from build123d import *

# Parameters (mm, degrees)
SKETCH1_W                       = 46
SKETCH1_H                       = 32
BOSS_EXTRUDE1_DEPTH             = 2
CBORE_FOR_M3_SBHCS1_AT_2_COUNT  = 2
CBORE_FOR_M3_SBHCS1_AT_2_PITCH  = 18.273746641
CBORE_FOR_M3_SBHCS1_AT_3_COUNT  = 2
CBORE_FOR_M3_SBHCS1_AT_3_PITCH  = 37.721741957
CBORE_FOR_M3_SBHCS1_AT_4_COUNT  = 2
CBORE_FOR_M3_SBHCS1_AT_4_PITCH  = 33
BOSS_EXTRUDE2_START             = 3.63
SKETCH9_R                       = 3.35
SKETCH9_R_2                     = 1.7
BOSS_EXTRUDE2_DEPTH             = 3.63
SKETCH11_R                      = 5
SKETCH11_R_2                    = 3
BOSS_EXTRUDE3_DEPTH             = 2
CBORE_FOR_M1_6_SHCS1_AT_2_COUNT = 2
CBORE_FOR_M1_6_SHCS1_AT_2_PITCH = 33.25
CBORE_FOR_M1_6_SHCS1_AT_3_COUNT = 2
CBORE_FOR_M1_6_SHCS1_AT_3_PITCH = 51.03253864
CBORE_FOR_M1_6_SHCS1_AT_4_COUNT = 2
CBORE_FOR_M1_6_SHCS1_AT_4_PITCH = 28.4
CUT_EXTRUDE1_START              = -2
SKETCH17_R                      = 3
CUT_EXTRUDE1_DEPTH              = 2
FILLET1_R                       = 1.5
SKETCH18_W                      = 2
SKETCH18_H                      = 24
BOSS_EXTRUDE4_DEPTH             = 17.5
SKETCH19_R                      = 1.215
SKETCH19_R_2                    = 1.22
BOSS_EXTRUDE5_DEPTH             = 17.5


with BuildPart() as part:
    # Sketch1 → Boss-Extrude1 (new body)
    with BuildSketch(Plane(origin=(0, 0, 0), x_dir=(1, 0, 0), z_dir=(0, 1, 0))):
        with Locations((-23, -16)):
            Rectangle(SKETCH1_W, SKETCH1_H)
    extrude(amount=BOSS_EXTRUDE1_DEPTH)

    # Sketch7 → CBORE for M3 SBHCS1 (revolve, cut)
    with BuildSketch(Plane(origin=(-39.5, 2, 6.726253359), x_dir=(0, 0, 1), z_dir=(1, 0, 0))):
        Polygon((0, 0), (0, 3.021463052), (1.7, 2), (1.7, 1.65), (3.35, 1.65), (3.35, 0.025), (3.375, 0), align=None)
    cbore_for_m3_sbhcs1 = revolve(axis=Axis((-39.5, 8.35, 6.726253359), (0, -1, 0)), mode=Mode.SUBTRACT)

    # CBORE for M3 SBHCS1 at 2: CBORE for M3 SBHCS1 ×2
    with Locations(*[(0, 0, i * CBORE_FOR_M3_SBHCS1_AT_2_PITCH) for i in range(1, CBORE_FOR_M3_SBHCS1_AT_2_COUNT)]):
        add(cbore_for_m3_sbhcs1, mode=Mode.SUBTRACT)

    # CBORE for M3 SBHCS1 at 3: CBORE for M3 SBHCS1 ×2
    with Locations(*[Vector(0.874827043707974, 0, 0.4844353864006702) * (i * CBORE_FOR_M3_SBHCS1_AT_3_PITCH) for i in range(1, CBORE_FOR_M3_SBHCS1_AT_3_COUNT)]):
        add(cbore_for_m3_sbhcs1, mode=Mode.SUBTRACT)

    # CBORE for M3 SBHCS1 at 4: CBORE for M3 SBHCS1 ×2
    with Locations(*[(i * CBORE_FOR_M3_SBHCS1_AT_4_PITCH, 0, 0) for i in range(1, CBORE_FOR_M3_SBHCS1_AT_4_COUNT)]):
        add(cbore_for_m3_sbhcs1, mode=Mode.SUBTRACT)

    # Sketch9 → Boss-Extrude2 (add)
    # profile 1 of 4: a face of its own
    with BuildSketch(Plane(origin=(-49.887058416, 0.35, -0.273746641), x_dir=(1, 0, 0), z_dir=(0, 1, 0)).offset(BOSS_EXTRUDE2_START)):
        with Locations(Location((10.387058416, -25.273746641, 0), (0, 0, 90))):
            Circle(SKETCH9_R)
        with Locations(Location((10.387058416, -25.273746641, 0), (0, 0, 270))):
            Circle(SKETCH9_R_2, mode=Mode.SUBTRACT)
    # profile 2 of 4: a face of its own
    with BuildSketch(Plane(origin=(-49.887058416, 0.35, -0.273746641), x_dir=(1, 0, 0), z_dir=(0, 1, 0)).offset(BOSS_EXTRUDE2_START)):
        with Locations(Location((43.387058416, -25.273746641, 0), (0, 0, 90))):
            Circle(SKETCH9_R)
        with Locations(Location((43.387058416, -25.273746641, 0), (0, 0, 270))):
            Circle(SKETCH9_R_2, mode=Mode.SUBTRACT)
    # profile 3 of 4: a face of its own
    with BuildSketch(Plane(origin=(-49.887058416, 0.35, -0.273746641), x_dir=(1, 0, 0), z_dir=(0, 1, 0)).offset(BOSS_EXTRUDE2_START)):
        with Locations(Location((43.387058416, -7, 0), (0, 0, 90))):
            Circle(SKETCH9_R)
        with Locations(Location((43.387058416, -7, 0), (0, 0, 270))):
            Circle(SKETCH9_R_2, mode=Mode.SUBTRACT)
    # profile 4 of 4: a face of its own
    with BuildSketch(Plane(origin=(-49.887058416, 0.35, -0.273746641), x_dir=(1, 0, 0), z_dir=(0, 1, 0)).offset(BOSS_EXTRUDE2_START)):
        with Locations(Location((10.387058416, -7, 0), (0, 0, 90))):
            Circle(SKETCH9_R)
        with Locations(Location((10.387058416, -7, 0), (0, 0, 270))):
            Circle(SKETCH9_R_2, mode=Mode.SUBTRACT)
    extrude(amount=-BOSS_EXTRUDE2_DEPTH)

    # Sketch11 → Boss-Extrude3 (add)
    with BuildSketch(Plane(origin=(-49.887058416, 2, -0.273746641), x_dir=(1, 0, 0), z_dir=(0, 1, 0))):
        with Locations(Location((19.387058416, -16, 0), (0, 0, 270))):
            Circle(SKETCH11_R)
        with Locations(Location((19.387058416, -16, 0), (0, 0, 270))):
            Circle(SKETCH11_R_2, mode=Mode.SUBTRACT)
    extrude(amount=BOSS_EXTRUDE3_DEPTH)

    # Sketch16 → CBORE for M1.6 SHCS1 (revolve, cut)
    with BuildSketch(Plane(origin=(-44.2, 2, 1.8), x_dir=(0, 0, 1), z_dir=(1, 0, 0))):
        Polygon((0, 0), (0, 2), (0.9, 2), (0.9, 1.6), (1.75, 1.6), (1.75, 0.025), (1.775, 0), align=None)
    cbore_for_m1_6_shcs1 = revolve(axis=Axis((-44.2, 8.35, 1.8), (0, -1, 0)), mode=Mode.SUBTRACT)

    # CBORE for M1.6 SHCS1 at 2: CBORE for M1.6 SHCS1 ×2
    with Locations(*[(i * CBORE_FOR_M1_6_SHCS1_AT_2_PITCH, 0, 0) for i in range(1, CBORE_FOR_M1_6_SHCS1_AT_2_COUNT)]):
        add(cbore_for_m1_6_shcs1, mode=Mode.SUBTRACT)

    # CBORE for M1.6 SHCS1 at 3: CBORE for M1.6 SHCS1 ×2
    with Locations(*[Vector(0.8308424611100395, 0, 0.5565076862152155) * (i * CBORE_FOR_M1_6_SHCS1_AT_3_PITCH) for i in range(1, CBORE_FOR_M1_6_SHCS1_AT_3_COUNT)]):
        add(cbore_for_m1_6_shcs1, mode=Mode.SUBTRACT)

    # CBORE for M1.6 SHCS1 at 4: CBORE for M1.6 SHCS1 ×2
    with Locations(*[(0, 0, i * CBORE_FOR_M1_6_SHCS1_AT_4_PITCH) for i in range(1, CBORE_FOR_M1_6_SHCS1_AT_4_COUNT)]):
        add(cbore_for_m1_6_shcs1, mode=Mode.SUBTRACT)

    # Sketch17 → Cut-Extrude1 (cut)
    with BuildSketch(Plane(origin=(0, 2, 0), x_dir=(1, 0, 0), z_dir=(0, 1, 0)).offset(CUT_EXTRUDE1_START)):
        with Locations(Location((-30.5, -15.726253359, 0), (0, 0, 270))):
            Circle(SKETCH17_R)
    extrude(amount=CUT_EXTRUDE1_DEPTH, mode=Mode.SUBTRACT)

    # Fillet1
    fillet1_edges = [part.edges().sort_by_distance(p)[0] for p in [
        (0, 1, 32),
        (0, 1, 0),
        (-46, 1, 0),
        (-46, 1, 32),
    ]]
    fillet(fillet1_edges, radius=FILLET1_R)

    # Sketch18 → Boss-Extrude4 (add)
    with BuildSketch(Plane.XZ):
        with Locations((-45, 16)):
            Rectangle(SKETCH18_W, SKETCH18_H)
    extrude(amount=BOSS_EXTRUDE4_DEPTH)

    # Sketch19 → Boss-Extrude5 (add)
    with BuildSketch(Plane.XZ):
        with Locations(Location((-18.516057742, 22.467738948, 0), (0, 0, 90))):
            Circle(SKETCH19_R)
        with Locations(Location((-8.600917975, 21.167737636, 0), (0, 0, 90))):
            Circle(SKETCH19_R_2)
    extrude(amount=BOSS_EXTRUDE5_DEPTH)


solid = part.part
Part model, mm, in its own coordinate system. A direction names the side the tool comes from. Coordinates: 2 decimals unless noted, no trailing zeros. Order: outer loops, then holes, each group sorted by start corner. A loop starts at its lowest first (then second) coordinate and runs counter-clockwise, first axis right, second up. Notation, with made-up numbers: (21, 59) - (79, 59) arc R18 ccw to (79, 90) - close; hole circle Ø9 at (-8, 69.25). An arc over 180 degrees is marked (long way). Use CSV: the item, a comma, the result in double quotes.
Item 1: Probe probe 1 along Z at (x, y) = (-44.2, 0.2); probe 2 along Z at (x, y) = (-39.5, 0.1); probe 3 along X at (y, z) = (0.35, 25). List the from-to ranges inside material, lowest first.
Solved:
probe 1,"z = 0 to 0.9, 2.7 to 29.3, 31.1 to 32"
probe 2,"z = 0 to 5.03, 8.43 to 23.3, 26.7 to 32"
probe 3,"x = -46 to -41.2, -37.8 to -8.2, -4.8 to 0"
Item 2: Saw through at B-B on y = 2.5. Give the number of separate pieces and of enclosed holes in the cut face, and give its area (3 significant figures).
Solved:
separate pieces,"5"
enclosed holes,"5"
area,"155 mm²"
Item 3: Saw through at A-A on x = -6.5. Give the cut face in (y, z) (3 decimals), and give its area (3 significant figures).
Solved:
outline,"(0, 0) - (2, 0) - (2, 3.351) - (1.975, 3.376) - (3.98, 3.376) - (3.98, 5.026) - (0, 5.026) - close; (0, 8.426) - (3.98, 8.426) - (3.98, 10.076) - (1.975, 10.076) - (2, 10.101) - (2, 21.625) - (1.975, 21.65) - (3.98, 21.65) - (3.98, 23.3) - (0, 23.3) - close; (0, 26.7) - (3.98, 26.7) - (3.98, 28.35) - (1.975, 28.35) - (2, 28.375) - (2, 32) - (0, 32) - close"
area,"63.5 mm²"
Item 4: Saw through at C-C on z = 25. Give the cut face in (x, y) (3 decimals).
Solved:
outline,"(-46, -17.5) - (-44, -17.5) - (-44, 0) - (-41.2, 0) - (-41.2, 3.98) - (-42.85, 3.98) - (-42.85, 1.975) - (-42.875, 2) - (-46, 2) - close; (-37.8, 0) - (-8.2, 0) - (-8.2, 3.98) - (-9.85, 3.98) - (-9.85, 1.975) - (-9.875, 2) - (-36.125, 2) - (-36.15, 1.975) - (-36.15, 3.98) - (-37.8, 3.98) - close; (-4.8, 0) - (0, 0) - (0, 2) - (-3.125, 2) - (-3.15, 1.975) - (-3.15, 3.98) - (-4.8, 3.98) - close"
Item 5: Mould opens along X. For faces 3 (the face through (-33, 4, 18)), 4 (the face through (-45, 0.4, 31)), 5 (the face through (-0.45, 1.01, 31.57)), 6 (the face through (-7.506, 2.992, 21.805)) say: +X half, -X half, draft (parallel to the pull), parting line (faces both ways), or undercut.
Solved:
face 3,"draft"
face 4,"undercut"
face 5,"+X half"
face 6,"undercut"
Item 6: Saw through at D-D on y = -5.75. Give the cut face in (x, z) (3 decimals).
Solved:
outline,"(-46, 4) - (-44, 4) - (-44, 28) - (-46, 28) - close; circle Ø2.43 at (-18.516, 22.468); circle Ø2.44 at (-8.601, 21.168)"
Item 7: Drop flat-ended pins along their axis: P1, Ø3, axis at x = -9, y = -3.5, coming from the -Z side; P2, Ø6, axis at x = -11.5, z = 11, coming from the -Y side; P3, Ø2, axis at x = -4.5, z = 27.5, coming from the +Y side; P4, Ø9.5, axis at x = -12, z = 20.5, coming from the -Y side. Give the stop position or say it passes through.
Solved:
P1,"stops at z = 19.95"
P2,"stops at y = 0"
P3,"stops at y = 3.98"
P4,"stops at y = -17.5"
Item 8: 3-axis set-ups, long thin cutter, end or side, ignore diameter. For faces 1 (the face through (-12.426, 1.199, 2.741)), 2 (the face through (-10.152, 0.203, 2.215)): which of +Z, -Z, +X, -X, +Y, -Y reach the whole face in a straight line?
Solved:
face 1,"+Y"
face 2,"+Y, -Y"
